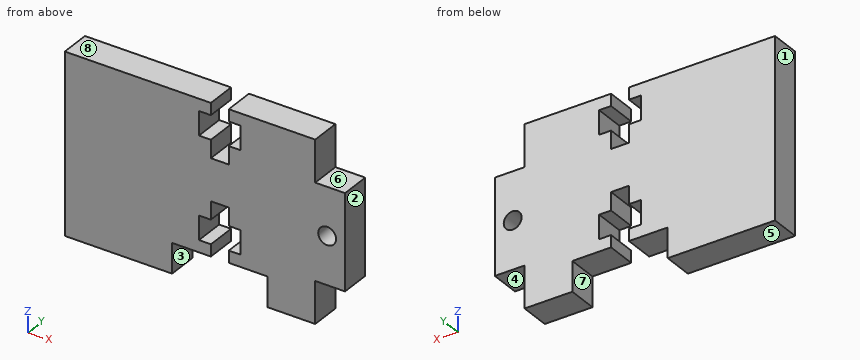
from build123d import *

# Parameters (mm, degrees)
CROQUIS1_W              = 32
CROQUIS1_H              = 30
SALIENTE_EXTRUIR1_DEPTH = 5
CORTAR_EXTRUIR1_DEPTH   = 23.494443758
CORTAR_EXTRUIR2_DEPTH   = 23.494443758
CROQUIS4_W              = 10
CROQUIS4_H              = 16
SALIENTE_EXTRUIR2_DEPTH = 5
CROQUIS5_R              = 1.5
CORTAR_EXTRUIR3_DEPTH   = 27.286878856
CROQUIS6_W              = 10
CROQUIS6_H              = 30
SALIENTE_EXTRUIR3_DEPTH = 5


with BuildPart() as part:
    # Croquis1 → Saliente-Extruir1 (new body)
    with BuildSketch(Plane(origin=(0, 0, 0), x_dir=(1, 0, 0), z_dir=(0, 1, 0))):
        Rectangle(CROQUIS1_W, CROQUIS1_H)
    extrude(amount=SALIENTE_EXTRUIR1_DEPTH)

    # Croquis2 → Cortar-Extruir1 (cut, through all)
    with BuildSketch(Plane(origin=(0, 5, 0), x_dir=(1, 0, 0), z_dir=(0, 1, 0))):
        Polygon((-8, 15), (8, 15), (8, 10), (1.5, 10), (1.5, 8), (3.5, 8), (3.5, 4), (1.5, 4), (1.5, 1), (-1.5, 1), (-1.5, 4), (-3.5, 4), (-3.5, 8), (-1.5, 8), (-1.5, 10), (-8, 10), align=None)
    extrude(amount=-CORTAR_EXTRUIR1_DEPTH, mode=Mode.SUBTRACT)

    # Croquis3 → Cortar-Extruir2 (cut, through all)
    with BuildSketch(Plane(origin=(0, 5, 0), x_dir=(1, 0, 0), z_dir=(0, 1, 0))):
        Polygon((1.5, -15), (1.5, -13), (3.5, -13), (3.5, -9), (1.5, -9), (1.5, -6), (-1.5, -6), (-1.5, -9), (-3.5, -9), (-3.5, -13), (-1.5, -13), (-1.5, -15), align=None)
    extrude(amount=-CORTAR_EXTRUIR2_DEPTH, mode=Mode.SUBTRACT)

    # Croquis4 → Saliente-Extruir2 (add)
    with BuildSketch(Plane(origin=(0, 5, 0), x_dir=(1, 0, 0), z_dir=(0, 1, 0))):
        with Locations((16, 0)):
            Rectangle(CROQUIS4_W, CROQUIS4_H)
    extrude(amount=-SALIENTE_EXTRUIR2_DEPTH)

    # Croquis5 → Cortar-Extruir3 (cut, through all)
    with BuildSketch(Plane(origin=(0, 5, 0), x_dir=(1, 0, 0), z_dir=(0, 1, 0))):
        with Locations(Location((18, 0, 0), (0, 0, 270))):
            Circle(CROQUIS5_R)
    extrude(amount=-CORTAR_EXTRUIR3_DEPTH, mode=Mode.SUBTRACT)

    # Croquis6 → Saliente-Extruir3 (add)
    with BuildSketch(Plane(origin=(0, 5, 0), x_dir=(1, 0, 0), z_dir=(0, 1, 0))):
        with Locations((-21, 0)):
            Rectangle(CROQUIS6_W, CROQUIS6_H)
    extrude(amount=-SALIENTE_EXTRUIR3_DEPTH)


solid = part.part
The model under review builds one solid part; all positions refer to its coordinate system, in mm. Face numbers are marked on the shaded views. A direction names the side the tool comes from. Round coordinates to 2 decimals unless told otherwise and drop trailing zeros. Order: outer loops, then holes, each group sorted by start corner. A loop starts at its lowest first (then second) coordinate and runs counter-clockwise, first axis right, second up. Notation, with made-up numbers: (-37.5, 33) -> (14.5, 33) arc R17 cw to (14.5, 48) -> close; hole circle Ø3 at (45.25, 26). An arc over 180 degrees is marked (long way). Use CSV: the item, a comma, the result in double quotes. Start each with the question number.
(1) Consider section B-B on x = 18. Write out the cut boundary in (y, z), and give its area (3 significant figures).
(2) Mouldability with a two-part tool opening along X and no side actions: class the marked faces 1, 2 and 3 as pulls with the +X half, pulls with the -X half, needs draft (parallel to the pull), parting line crosses it, or undercut.
(3) Tool access review of the marked faces 4, 5, 6, 7 and 8: name each direction out of +Z, -Z, +X, -X, +Y, -Y from which nothing blocks a thin tool from reaching the whole face with its end or side.
(4) Wall thickness on probe 1 along Z at (x, y) = (2.5, 1.15); probe 2 along X at (y, z) = (2.35, 8.5); probe 3 along X at (y, z) = (3.6, 0): over which ranges is each line inside the solid? List them lowest first. Write a range as from..to.
(5) Insertion check: pin 1 (1 mm diameter, centred on x = 2.5, y = 2, fed in from -Z); pin 2 (2 mm diameter, centred on y = 3, z = 14.5, fed in from +X); pin 3 (1.5 mm diameter, centred on x = -0.5, y = 2, fed in from -Z). Each pin has a flat end and moves straight along its axis. Give the tip position at first contact, or say it passes through.
(6) Consider section C-C on x = 0. Write out the cut boundary in (y, z), and give its area (3 significant figures).
(7) Consider section A-A on z = -7.5. Write out the cut boundary in (x, y), and give its area (3 significant figures).
Responses:
1,outline,"(0, -8) -> (5, -8) -> (5, -1.5) -> (0, -1.5) -> close; (0, 1.5) -> (5, 1.5) -> (5, 8) -> (0, 8) -> close"
1,area,"65.0 mm²"
2,face 1,"pulls with the -X half"
2,face 2,"pulls with the +X half"
2,face 3,"undercut"
3,face 4,"-Z, +X, +Y, -Y"
3,face 5,"-Z, +X, -X, +Y, -Y"
3,face 6,"+Z, +X, +Y, -Y"
3,face 7,"-Z, +Y, -Y"
3,face 8,"+Z, +X, -X, +Y, -Y"
4,probe 1,"-10..-8, -4..9, 13..15"
4,probe 2,"-26..-1.5, 1.5..16"
4,probe 3,"-26..16.5, 19.5..21"
5,pin 1,"z = -10"
5,pin 2,"x = 16"
5,pin 3,"z = -1"
6,outline,"(0, -1) -> (5, -1) -> (5, 6) -> (0, 6) -> close"
6,area,"35.0 mm²"
7,outline,"(-26, 0) -> (-3.5, 0) -> (-3.5, 5) -> (-26, 5) -> close; (3.5, 0) -> (21, 0) -> (21, 5) -> (3.5, 5) -> close"
7,area,"200 mm²"
